Could you check a few things on this model? Use its own coordinates, in mm. Face numbers are marked on the shaded views. A direction names the side the tool comes from. Give positions to 0.01 mm unless a question says otherwise; leave off trailing zeros. Write each loop counter-clockwise with the first axis right and the second up, starting at its lowest first coordinate (ties: lowest second). Pieces come first, ordered by that corner, then holes. Notation, with made-up numbers: M 46.5,13.25 L 79.5,13.25 A19 ccw 79.5,41.25 Z; hole C -12.75,8 d7. An arc over 180 degrees is marked long. Answer as CSV lines item,"result". Start each with the question number.
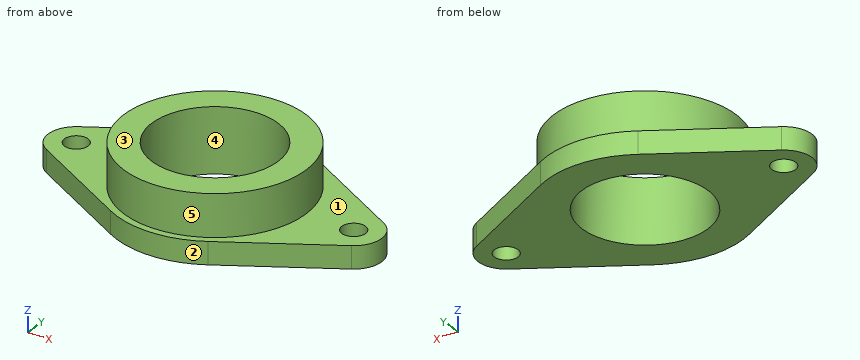
from build123d import *

# Parameters (mm, degrees)
SKETCH2_R           = 4.25
SKETCH2_R_2         = 32.5
BOSS_EXTRUDE1_DEPTH = 8
SKETCH2_4_R         = 32.5
SKETCH2_4_R_2       = 22.5
BOSS_EXTRUDE2_DEPTH = 23


with BuildPart() as part:
    # Sketch2 → Boss-Extrude1 (new body)
    with BuildSketch(Plane.XY):
        with BuildLine():
            Line((17.5, 30.310889132), (55, 8.660254038))
            ThreePointArc((55, 8.660254038), (60, 0), (55, -8.660254038))
            Line((55, -8.660254038), (17.5, -30.310889132))
            ThreePointArc((17.5, -30.310889132), (0, -35), (-17.5, -30.310889132))
            Line((-17.5, -30.310889132), (-55, -8.660254038))
            ThreePointArc((-55, -8.660254038), (-60, 0), (-55, 8.660254038))
            Line((-55, 8.660254038), (-17.5, 30.310889132))
            ThreePointArc((-17.5, 30.310889132), (0, 35), (17.5, 30.310889132))
        make_face()
        with Locations((50, 0)):
            Circle(SKETCH2_R, mode=Mode.SUBTRACT)
        with Locations((-50, 0)):
            Circle(SKETCH2_R, mode=Mode.SUBTRACT)
        Circle(SKETCH2_R_2, mode=Mode.SUBTRACT)
    extrude(amount=BOSS_EXTRUDE1_DEPTH)

    # Sketch2_4 → Boss-Extrude2 (add)
    with BuildSketch(Plane.XY):
        Circle(SKETCH2_4_R)
        Circle(SKETCH2_4_R_2, mode=Mode.SUBTRACT)
    extrude(amount=BOSS_EXTRUDE2_DEPTH)


solid = part.part
1. Please list where these lines run through material, in increasing order: line 1 (Y direction, x = 0, z = 16); line 2 (Z direction, x = 34, y = -14.5); line 3 (X direction, y = 8, z = 14).
2. Imagine slicing it at D-D, the plane y = -15.5. Please give me the cut outline in (x, z), plus the area to 3 significant figures.
3. On a 3-axis mill with a long thin cutter (end or side, diameter ignored), from which of +Z, -Z, +X, -X, +Y, -Y can I reach the whole of each face in a straight line? I mean the marked faces 1 and 2. Say none if no direction works.
4. Thinking about a two-plate mould opening in Y: for the marked faces 3, 4 and 5, which applies, pulls with the +Y half, pulls with the -Y half, needs draft (parallel to the pull), parting line crosses it, or undercut?
5. Will these pins go through, and if not, where does the flat tip stop? P1, Ø5, axis at y = -23, z = 19.5, coming from the -X side; P2, Ø5, axis at x = -26.5, z = 16.5, coming from the +Y side; P3, Ø4, axis at y = 9.5, z = 19, coming from the +X side.
6. Imagine slicing it at A-A, the plane x = 0. Please give me the cut outline in (y, z), plus the area to 3 significant figures.
7. Imagine slicing it at C-C, the plane z = 6.5. Please give me the cut outline in (x, y), plus the area to 3 significant figures.
8. Imagine slicing it at B-B, the plane y = 0. Please give me the cut outline in (x, z), plus the area to 3 significant figures.
Solutions:
1,line 1,"-32.5 to -22.5, 22.5 to 32.5"
1,line 2,"0 to 8"
1,line 3,"-31.5 to -21.03, 21.03 to 31.5"
2,outline,"M -43.15,0 L -16.31,0 L -16.31,23 L -28.57,23 L -28.57,8 L -43.15,8 Z; M 16.31,0 L 43.15,0 L 43.15,8 L 28.57,8 L 28.57,23 L 16.31,23 Z"
2,area,"797 mm²"
3,face 1,"+Z"
3,face 2,"+Z, -Z, -Y"
4,face 3,"needs draft"
4,face 4,"undercut"
4,face 5,"parting line crosses it"
5,P1,"x = -25.22"
5,P2,"y = 21.91"
5,P3,"x = 31.62"
6,outline,"M -35,0 L -22.5,0 L -22.5,23 L -32.5,23 L -32.5,8 L -35,8 Z; M 22.5,0 L 35,0 L 35,8 L 32.5,8 L 32.5,23 L 22.5,23 Z"
6,area,"500 mm²"
7,outline,"M -55,-8.66 L -17.5,-30.31 A35 ccw 17.5,-30.31 L 55,-8.66 A10 ccw 55,8.66 L 17.5,30.31 A35 ccw -17.5,30.31 L -55,8.66 A10 ccw Z; hole C -50,0 d8.5; hole C 0,0 d45; hole C 50,0 d8.5"
7,area,"3,690 mm²"
8,outline,"M -60,0 L -54.25,0 L -54.25,8 L -60,8 Z; M -45.75,0 L -22.5,0 L -22.5,23 L -32.5,23 L -32.5,8 L -45.75,8 Z; M 22.5,0 L 45.75,0 L 45.75,8 L 32.5,8 L 32.5,23 L 22.5,23 Z; M 54.25,0 L 60,0 L 60,8 L 54.25,8 Z"
8,area,"764 mm²"
